Autodesk Inventor part; units mm, degrees
ref_plane "YZ Plane" through (0, 0, 0) normal (1, 0, 0) x (0, 1, 0)
ref_plane "XZ Plane" through (0, 0, 0) normal (0, 1, 0) x (-1, 0, 0)
ref_plane "XY Plane" through (0, 0, 0) normal (0, 0, 1) x (1, 0, 0)
sketch "スケッチ1" plane through (0, 0, 0) normal (0, 0, 1) x (1, 0, 0)
  circle A0 centre (0, 0) radius 4
  dimension "d0" = 8
extrude "押し出し1" add sketch "スケッチ1" along normal blind 1
sketch "スケッチ2" plane through (0, 0, 1) normal (0, 0, 1) x (1, 0, 0)
  circle A0 centre (0, 0) radius 1.5
  dimension "d3" = 3
hole "穴1" at (0, 0, 1) direction (0, 0, -1) diameter 3 end through all
chamfer "面取り1" distance 0.3 angle 45 1 edges at (0, 1.5, 1)
sketch "スケッチ3" plane through (0, 0, 0) normal (0, 0, -1) x (-1, 0, 0)
  circle A0 centre (0, 0) radius 1.5
  circle A1 centre (0, 0) radius 1.5
  circle A2 centre (0, 0) radius 2.5
  dimension "d14" = 5
extrude "押し出し2" add sketch "スケッチ3" along normal blind 5
properties part number "RD018_ブッシュ80F-0305"
Source: CAD feature listing. Evaluate the final solid. Frame: model axes, mm. A direction names the side the tool comes from. Round coordinates to 2 decimals unless told otherwise and drop trailing zeros. Loops run counter-clockwise (first coordinate to the right, second up) from the corner with the lowest first, then second, coordinate; pieces in that order, holes last.
1. Contact query for flat-ended pins moving along their axis: pin 1 (1 mm diameter, centred on x = 2, z = -3, fed in from -Y); pin 2 (2.5 mm diameter, centred on x = 0, y = 0, fed in from +Z); pin 3 (1 mm diameter, centred on x = 1, z = -2.5, fed in from +Y); pin 4 (2 mm diameter, centred on x = 1, z = 0, fed in from +Y). Output: stop coordinate, or through.
2. Section query D-D on x = 3.25. Output: boundary loops of the cut face in (y, z), and give its area (3 significant figures).
3. Access query for faces 1 (the flat face through (2, 2, 0)), 2 (the flat face through (-2, 0, -5)). Directions: +Z, -Z, +X, -X, +Y, -Y. A direction counts if a zero-diameter tool reaches every point of the face in a straight line with its end or side. Return the directions, or none.
4. Section query A-A on y = 0. Output: boundary loops of the cut face in (x, z), and give its area (3 significant figures).
5. Section query C-C on z = -1.85. Output: boundary loops of the cut face in (x, y), and give its area (3 significant figures).
6. Mould query, pull axis X, two halves, no side actions, for faces 3 (the flat face through (2, -1, 1)), 4 (the cylindrical face through (-0.867, 3.905, 0.493)), 5 (the cylindrical face through (-1.39, -0.56, -2.11)). Classes: released by +X, released by -X, zero draft, split by the parting line, or undercut.
7. Ray query, L1, parallel to Y at x = 0, z = -3.75; L2, parallel to Z at x = 3.5, y = -1; L3, parallel to X at y = 0.25, z = -3.7. Return the intervals inside material, ascending.
Answers below:
1. pin 1: stops at y = -2
1. pin 2: passes through
1. pin 3: stops at y = 2.45
1. pin 4: stops at y = 4
2. outline: (-2.33, 0) - (2.33, 0) - (2.33, 1) - (-2.33, 1) - close
2. area: 4.66 mm2
3. face 1: -Z
3. face 2: -Z, +X, -X, +Y, -Y
4. outline: (-4, 0) - (-2.5, 0) - (-2.5, -5) - (-1.5, -5) - (-1.5, 0.7) - (-1.8, 1) - (-4, 1) - close; (1.5, -5) - (2.5, -5) - (2.5, 0) - (4, 0) - (4, 1) - (1.8, 1) - (1.5, 0.7) - close
4. area: 14.9 mm2
5. outline: circle Ø5 at (0, 0); hole circle Ø3 at (0, 0)
5. area: 12.6 mm2
6. face 3: zero draft
6. face 4: split by the parting line
6. face 5: undercut
7. L1: y = -2.5 to -1.5, 1.5 to 2.5
7. L2: z = 0 to 1
7. L3: x = -2.49 to -1.48, 1.48 to 2.49
